Design review of the part shown in the three views and the two pictorial views. Dimensions are in mm from the part's minimum x, y and z. A direction names the side the tool comes from. Coordinates: 2 decimals unless noted, no trailing zeros. Write each loop counter-clockwise with the first axis right and the second up, starting at its lowest first coordinate (ties: lowest second). Pieces come first, ordered by that corner, then holes. Notation, with made-up numbers: (5.25, 51.25) - (52.25, 51.25) arc R36 ccw to (52.25, 88.25) - close; hole circle Ø11 at (13, 47). An arc over 180 degrees is marked (long way). Answer as CSV lines item,"result". Start each with the question number.
Q1. Machinability: for the marked faces 1 and 2, which of the approach directions +Z, -Z, +X, -X, +Y, -Y give a long, thin tool a straight path to every point of the face, cutting with its end or side? Answer none if there is none.
Q2. Clearance check with flat-ended pins moving along their axes: pin 1 (1 mm diameter, centred on x = 28, z = 23, fed in from +Y); pin 2 (1 mm diameter, centred on x = 37, z = 27, fed in from +Y); pin 3 (2 mm diameter, centred on x = 19.5, y = 27.5, fed in from -Z). State where each tip first meets the part, or that it passes through.
Q3. We need section A-A (z = 7). Write out the cut boundary in (x, y), plus the area to 3 significant figures.
Q4. For line 1 along X through (y, z) = (30, 6); line 2 along X through (y, z) = (30, 34), list the stretches that pass through material, from the lowest coordinate up. Write a range as [from, to].
Q5. Mouldability with a two-part tool opening along X and no side actions: class the marked faces 3, 4 and 5 as pulls with the +X half, pulls with the -X half, needs draft (parallel to the pull), parting line crosses it, or undercut.
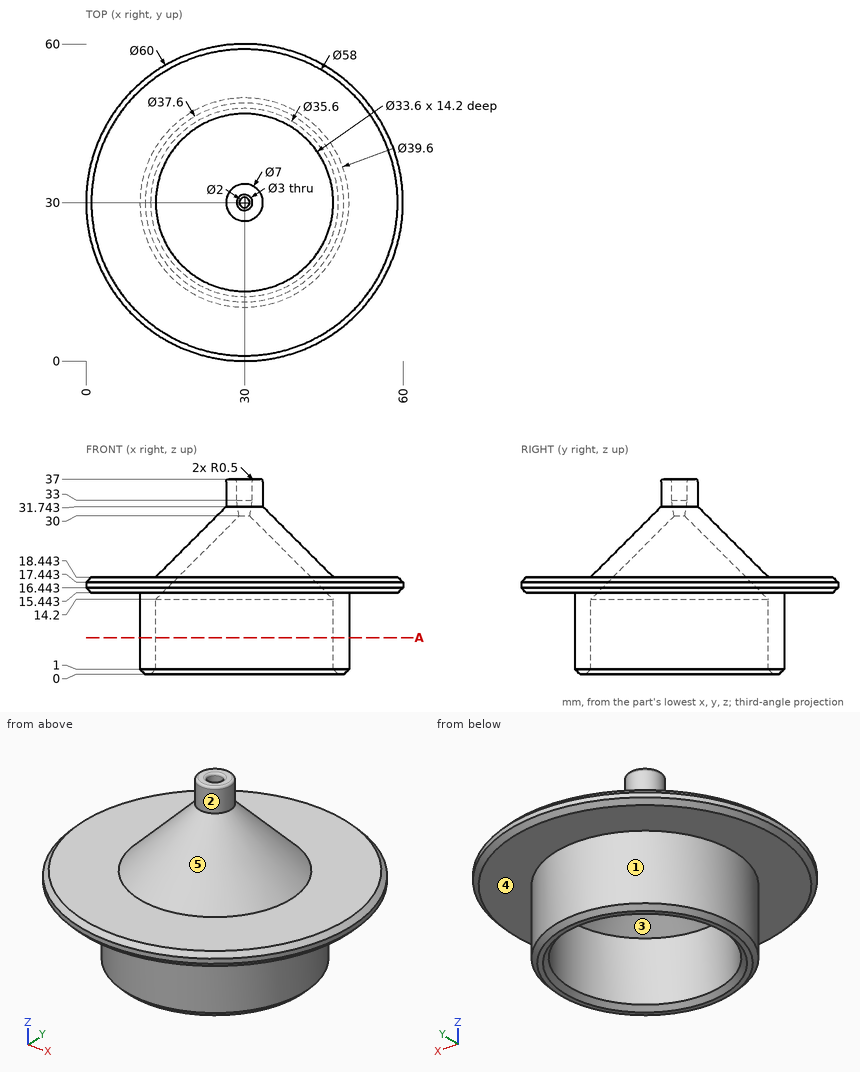
Results list:
1,face 1,"-Z"
1,face 2,"+Z"
2,pin 1,"stops at y = 42.59"
2,pin 2,"stops at y = 35.46"
2,pin 3,"stops at z = 19.21"
3,outline,"circle Ø39.6 at (30, 30); hole circle Ø33.6 at (30, 30)"
3,area,"345 mm2"
4,line 1,"x = [10.2, 13.2], [46.8, 49.8]"
4,line 2,"x = [26.5, 28.5], [31.5, 33.5]"
5,face 3,"undercut"
5,face 4,"needs draft"
5,face 5,"parting line crosses it"
